Part model, mm, in its own coordinate system. Give positions to 0.01 mm unless a question says otherwise; leave off trailing zeros.
1. Drop flat-ended pins along their axis: pin 1 Ø1.9 at (x, z) = (-9, 161.5) entering from +Y; pin 2 Ø1.9 at (x, z) = (-8, 139) entering from -Y; pin 3 Ø0.7 at (y, z) = (2, 129.5) entering from +X. Give the stop position or say it passes through.
2. Probe line 1 (Y direction, x = 5, z = 57); line 2 (X direction, y = -6.5, z = 19.5); line 3 (X direction, y = -7, z = 71.5). List the from-to ranges inside material, lowest first.
3. Slice it at A-A on z = 156.5. Give the number of separate pieces and of enclosed holes in the cut face, and give its area (3 significant figures).
from build123d import *

# Parameters (mm, degrees)
SKETCH1_R           = 2
BOSS_EXTRUDE1_DEPTH = 400


with BuildPart() as part:
    # Sketch1 → Boss-Extrude1 (new body)
    with BuildSketch(Plane.XY):
        Polygon((-5.389620664, 10), (5.389620664, 10), (6.9, 8.2), (4.5, 8.2), (4.5, 6.556171609), (7.151917065, 3.899773171), (9.480384758, 3.899773171), (10, 3.599773171), (10.519615242, 3.899773171), (12.848082935, 3.899773171), (15.5, 6.556171609), (15.5, 8.2), (13.1, 8.2), (14.610379336, 10), (20, 10), (20, 4.610379336), (18.2, 3.1), (18.2, 5.5), (16.556171609, 5.5), (13.9, 2.839339828), (13.9, 0.519615231), (13.599999981, 0), (13.9, -0.519615231), (13.9, -2.839339828), (16.556171609, -5.5), (18.2, -5.5), (18.2, -3.1), (20, -4.610379336), (20, -10), (14.610379336, -10), (13.1, -8.2), (15.5, -8.2), (15.5, -6.556171609), (12.839339828, -3.9), (10.519222362, -3.9), (10, -3.600226829), (9.480777638, -3.9), (7.160660172, -3.9), (4.5, -6.556171609), (4.5, -8.2), (6.9, -8.2), (5.389620664, -10), (-5.389620664, -10), (-6.9, -8.2), (-4.5, -8.2), (-4.5, -6.556171609), (-7.160432959, -3.900226829), (-9.480384758, -3.900226829), (-10, -3.600226829), (-10.519615242, -3.900226829), (-12.839339828, -3.9), (-15.5, -6.556171609), (-15.5, -8.2), (-13.1, -8.2), (-14.610379336, -10), (-20, -10), (-20, -4.610379336), (-18.2, -3.1), (-18.2, -5.5), (-16.556171609, -5.5), (-13.9, -2.839339828), (-13.9, -0.519615231), (-13.599999981, 0), (-13.9, 0.519615231), (-13.9, 2.839339828), (-16.556171609, 5.5), (-18.2, 5.5), (-18.2, 3.1), (-20, 4.610379336), (-20, 10), (-14.610379336, 10), (-13.1, 8.2), (-15.5, 8.2), (-15.5, 6.556171609), (-12.839339828, 3.9), (-10.519615242, 3.899773171), (-10, 3.599773171), (-9.480384758, 3.899773171), (-7.160660172, 3.9), (-4.5, 6.556171609), (-4.5, 8.2), (-6.9, 8.2), align=None)
        with Locations((-10, 0)):
            Circle(SKETCH1_R, mode=Mode.SUBTRACT)
        with Locations((10, 0)):
            Circle(SKETCH1_R, mode=Mode.SUBTRACT)
        Polygon((-6.1, -2.839339828), (-2.376887287, -6.556171609), (-2.376887287, -8.2), (2.376887287, -8.2), (2.376887287, -6.556171609), (6.1, -2.839339828), (6.1, 2.839339828), (2.383168219, 6.556171609), (2.383168219, 8.2), (-2.383168219, 8.2), (-2.383168219, 6.556171609), (-6.1, 2.839339828), align=None, mode=Mode.SUBTRACT)
    extrude(amount=BOSS_EXTRUDE1_DEPTH)


solid = part.part
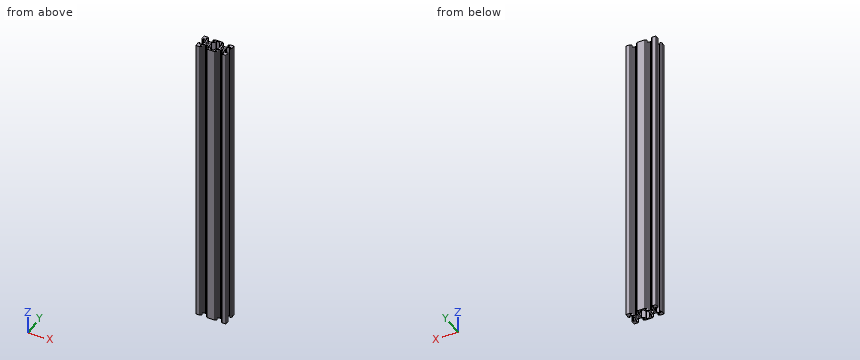
Data:
1. pin 1: stops at y = 3.9
1. pin 2: stops at y = -4.01
1. pin 3: stops at x = 13.9
2. line 1: y = -10 to -8.2, -6.06 to -3.94, 3.94 to 6.06, 8.2 to 10
2. line 2: x = -20 to -15.44, -4.56 to -2.43, 2.43 to 4.56, 15.44 to 20
2. line 3: x = -20 to -15.5, -4.5 to -2.38, 2.38 to 4.5, 15.5 to 20
3. separate pieces: 1
3. enclosed holes: 3
3. area: 301 mm2
